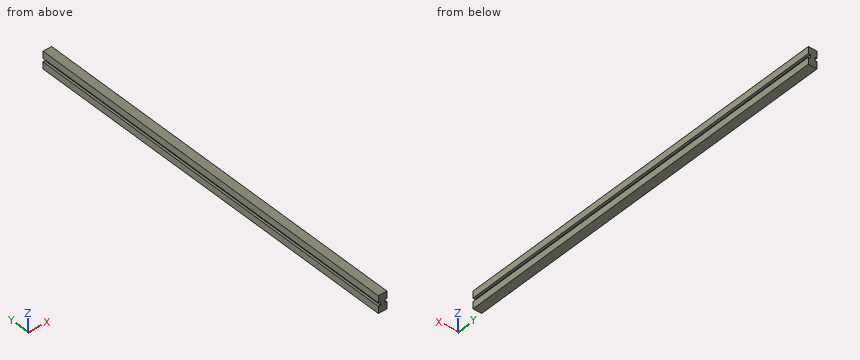
```python
from build123d import *

# Parameters (mm, degrees)
F1_DEPTH      = 400
F1_DEPTH_BACK = 500


with BuildPart() as f1:
    # F0 (on Front) → F1 (new body, two sides)
    with BuildSketch(Plane.XZ) as f1_sk:
        Polygon((-10, -20), (10, -20), (10, -4), (5, -4), (5, 4), (10, 4), (10, 20), (-10, 20), (-10, 4), (-5, 4), (-5, -4), (-10, -4), align=None)
    extrude(amount=F1_DEPTH)
    extrude(f1_sk.sketch, amount=-F1_DEPTH_BACK)


solid = f1.part
```
Check sheet for the modelled part. Datum: model origin and axes. Units: mm. Coordinates: 2 decimals unless noted, no trailing zeros. Loops run counter-clockwise (first coordinate to the right, second up) from the corner with the lowest first, then second, coordinate; pieces in that order, holes last. Notation, with made-up numbers: M 59.25,66 L 63.25,66 A31 ccw 63.25,100 Z; hole C 0,39.25 d2. An arc over 180 degrees is marked long. Answer as a JSON object with one key per item and string values.
1. Depth check by flat-ended pin: P1, Ø6.5, axis at y = -10, z = -1, coming from the -X side; P2, Ø6.5, axis at y = -70.5, z = 0.5, coming from the +X side. Enter the tip coordinate at first touch or a pass-through.
Outcome:
{"P1": "x = -10", "P2": "x = 5"}
2. Scan lines: L1, parallel to Z at x = 6.5, y = 245.5; L2, parallel to X at y = 137.5, z = 2.5. Record each from-to range of solid material in increasing order. Write a range as from..to.
Outcome:
{"L1": "-20..-4, 4..20", "L2": "-5..5"}
3. Sectioned sample at A-A on y = -285. Record the cut outline in (x, z), and give its area (3 significant figures).
Outcome:
{"outline": "M -10,-20 L 10,-20 L 10,-4 L 5,-4 L 5,4 L 10,4 L 10,20 L -10,20 L -10,4 L -5,4 L -5,-4 L -10,-4 Z", "area": "720 mm²"}
